Geometry check sheet. Reference: the model listing, model coordinates, mm. Face numbers are marked on the shaded views. A direction names the side the tool comes from. Give positions to 0.01 mm unless a question says otherwise; leave off trailing zeros. Order: outer loops, then holes, each group sorted by start corner. A loop starts at its lowest first (then second) coordinate and runs counter-clockwise, first axis right, second up. Notation, with made-up numbers: M 34.25,-1 L 92.25,-1 A22 cw 92.25,12 Z; hole C 38.5,-29 d6. An arc over 180 degrees is marked long. Put each result on its own line as item: value. Start each with the question number.
Q1. Material ranges on L1, parallel to X at y = -2.8, z = -135.5; L2, parallel to Z at x = 66.5, y = -4.25; L3, parallel to X at y = -14, z = -90, recorded low to high.
Q2. Section check B-B on z = -128.5. Record the cut outline in (x, y), then the cut area to 3 significant figures.
Q3. Access from +Z, -Z, +X, -X, +Y, -Y to the whole of each face (thin tool, end or side, straight path). Record for the marked faces 3 and 4.
Q4. Section check A-A on y = -12.5. Record the cut outline in (x, z).
Q5. Go/stop test with flat-tipped pins: pin 1 (1.6 mm diameter, centred on y = 1, z = -13.5, fed in from +X); pin 2 (3.5 mm diameter, centred on x = 94.5, z = -21, fed in from -Y); pin 3 (3.5 mm diameter, centred on x = 185, z = -22.5, fed in from -Y). Record where each tip stops, or that it passes through.
Q6. Mould release check, pull along X, two halves, no side actions. Record for the marked faces 1 and 2: +X half, -X half, draft (parallel to the pull), parting line (faces both ways), or undercut.
Q7. Section check C-C on z = -33. Record the cut outline in (x, y), then the cut area to 3 significant figures.
```python
from build123d import *

# Parameters (mm, degrees)
BOSS_EXTRUDE1_DEPTH     = 2
SKETCH2_W               = 45
SKETCH2_H               = 5
BOSS_EXTRUDE2_DEPTH     = 10
BOSS_EXTRUDE3_DEPTH     = 20
SKETCH4_W               = 67
SKETCH4_H               = 2
BOSS_EXTRUDE4_DEPTH     = 5
SKETCH5_W               = 58
SKETCH5_H               = 72.3
SKETCH5_W_2             = 55
SKETCH5_H_2             = 69.3
BOSS_EXTRUDE5_DEPTH     = 19
SKETCH6_W               = 13
SKETCH6_H               = 13
SKETCH6_W_2             = 10
CUT_EXTRUDE1_DEPTH      = 1.5
BOSS_EXTRUDE6_DEPTH     = 10
CUT_EXTRUDE2_START      = -6
SKETCH9_W               = 45
SKETCH9_H               = 1.5
CUT_EXTRUDE2_DEPTH      = 7
CUT_EXTRUDE3_DEPTH      = 12
SKETCH11_R              = 2.5
SKETCH11_R_2            = 1.5
BOSS_EXTRUDE7_DEPTH     = 4
SKETCH12_W              = 34
SKETCH12_H              = 63
SKETCH12_W_2            = 32
SKETCH12_H_2            = 61
BOSS_EXTRUDE8_DEPTH     = 4
SKETCH13_W              = 8
SKETCH13_H              = 4
CUT_EXTRUDE4_DEPTH      = 18
SKETCH14_R              = 6
SKETCH14_W              = 64
SKETCH14_H              = 39
CUT_EXTRUDE5_DEPTH      = 21
CUT_EXTRUDE5_DEPTH_BACK = 3
SKETCH15_W              = 100
SKETCH15_H              = 3
SKETCH15_W_2            = 112
BOSS_EXTRUDE9_DEPTH     = 5
CUT_EXTRUDE6_DEPTH      = 5


with BuildPart() as part:
    # Sketch1 → Boss-Extrude1 (new body)
    with BuildSketch(Plane(origin=(0, 0, 0), x_dir=(1, 0, 0), z_dir=(0, 1, 0))):
        with BuildLine():
            Line((124.25, 158), (176, 158))
            ThreePointArc((176, 158), (189.435028843, 152.435028843), (195, 139))
            Line((195, 139), (195, 19))
            ThreePointArc((195, 19), (189.435028843, 5.564971157), (176, 0))
            Line((176, 0), (162, 0))
            Line((162, 0), (162, 17))
            Line((162, 17), (120, 17))
            Line((120, 17), (120, 0))
            Line((120, 0), (75, 0))
            Line((75, 0), (75, 17))
            Line((75, 17), (33, 17))
            Line((33, 17), (33, 0))
            Line((33, 0), (19, 0))
            ThreePointArc((19, 0), (5.564971157, 5.564971157), (0, 19))
            Line((0, 19), (0, 139))
            ThreePointArc((0, 139), (5.564971157, 152.435028843), (19, 158))
            Line((19, 158), (70.75, 158))
            Line((70.75, 158), (70.75, 143))
            Line((70.75, 143), (80.75, 143))
            Line((80.75, 143), (80.75, 88))
            Line((80.75, 88), (114.25, 88))
            Line((114.25, 88), (114.25, 143))
            Line((114.25, 143), (124.25, 143))
            Line((124.25, 143), (124.25, 158))
        make_face()
    extrude(amount=BOSS_EXTRUDE1_DEPTH)

    # Sketch2 → Boss-Extrude2 (add)
    with BuildSketch(Plane.XZ):
        with Locations((97.5, -2.5)):
            Rectangle(SKETCH2_W, SKETCH2_H)
        with BuildLine():
            Line((33, 0), (33, -5))
            Line((33, -5), (19, -5))
            ThreePointArc((19, -5), (9.100505063, -9.100505063), (5, -19))
            Line((5, -19), (5, -139))
            ThreePointArc((5, -139), (9.100505063, -148.899494937), (19, -153))
            Line((19, -153), (70.75, -153))
            Line((70.75, -153), (70.75, -158))
            Line((70.75, -158), (19, -158))
            ThreePointArc((19, -158), (5.564971157, -152.435028843), (0, -139))
            Line((0, -139), (0, -19))
            ThreePointArc((0, -19), (5.564971157, -5.564971157), (19, 0))
            Line((19, 0), (33, 0))
        make_face()
        with BuildLine():
            Line((162, 0), (162, -5))
            Line((162, -5), (176, -5))
            ThreePointArc((176, -5), (185.899494937, -9.100505063), (190, -19))
            Line((190, -19), (190, -139))
            ThreePointArc((190, -139), (185.899494937, -148.899494937), (176, -153))
            Line((176, -153), (124.25, -153))
            Line((124.25, -153), (124.25, -158))
            Line((124.25, -158), (176, -158))
            ThreePointArc((176, -158), (189.435028843, -152.435028843), (195, -139))
            Line((195, -139), (195, -19))
            ThreePointArc((195, -19), (189.435028843, -5.564971157), (176, 0))
            Line((176, 0), (162, 0))
        make_face()
    extrude(amount=BOSS_EXTRUDE2_DEPTH)

    # Sketch3 → Boss-Extrude3 (add)
    with BuildSketch(Plane.XZ):
        Polygon((190, -43.5), (150, -43.5), (150, -114.5), (190, -114.5), (190, -112.5), (152, -112.5), (152, -45.5), (190, -45.5), align=None)
    extrude(amount=BOSS_EXTRUDE3_DEPTH)

    # Sketch4 → Boss-Extrude4 (add)
    with BuildSketch(Plane(origin=(152, 0, 0), x_dir=(0, 0, -1), z_dir=(1, 0, 0))):
        with Locations((79, -19)):
            Rectangle(SKETCH4_W, SKETCH4_H)
    extrude(amount=BOSS_EXTRUDE4_DEPTH)

    # Sketch5 → Boss-Extrude5 (add)
    with BuildSketch(Plane.XZ):
        with Locations((41.75, -116.85)):
            Rectangle(SKETCH5_W, SKETCH5_H)
        with Locations((41.75, -116.85)):
            Rectangle(SKETCH5_W_2, SKETCH5_H_2, mode=Mode.SUBTRACT)
    extrude(amount=BOSS_EXTRUDE5_DEPTH)

    # Sketch6 → Cut-Extrude1 (cut)
    with BuildSketch(Plane.XY.offset(-80.7)):
        with Locations((52.25, -9.5)):
            Rectangle(SKETCH6_W, SKETCH6_H)
        with Locations((20.75, -9.5)):
            Rectangle(SKETCH6_W_2, SKETCH6_H)
    extrude(amount=-CUT_EXTRUDE1_DEPTH, mode=Mode.SUBTRACT)

    # Sketch8 → Boss-Extrude6 (add, symmetric)
    with BuildSketch(Plane(origin=(29.25, 0, 0), x_dir=(0, 0, -1), z_dir=(1, 0, 0))):
        Polygon((151.5, -3.5), (150.5, -3.5), (151.5, -9.5), align=None)
    extrude(amount=BOSS_EXTRUDE6_DEPTH, both=True)

    # Sketch9 → Cut-Extrude2 (cut, through all)
    with BuildSketch(Plane.XZ.offset(10).offset(CUT_EXTRUDE2_START)):
        with BuildLine():
            ThreePointArc((0, -139), (5.564971157, -152.435028843), (19, -158))
            Line((19, -158), (70.75, -158))
            Line((70.75, -158), (70.75, -156.5))
            Line((70.75, -156.5), (19, -156.5))
            ThreePointArc((19, -156.5), (6.625631329, -151.374368671), (1.5, -139))
            Line((1.5, -139), (1.5, -19))
            ThreePointArc((1.5, -19), (6.625631329, -6.625631329), (19, -1.5))
            Line((19, -1.5), (33, -1.5))
            Line((33, -1.5), (33, 0))
            Line((33, 0), (19, 0))
            ThreePointArc((19, 0), (5.564971157, -5.564971157), (0, -19))
            Line((0, -19), (0, -139))
        make_face()
        with BuildLine():
            ThreePointArc((193.5, -19), (188.374368671, -6.625631329), (176, -1.5))
            Line((176, -1.5), (162, -1.5))
            Line((162, -1.5), (162, 0))
            Line((162, 0), (176, 0))
            ThreePointArc((176, 0), (189.435028843, -5.564971157), (195, -19))
            Line((195, -19), (195, -139))
            ThreePointArc((195, -139), (189.435028843, -152.435028843), (176, -158))
            Line((176, -158), (124.25, -158))
            Line((124.25, -158), (124.25, -156.5))
            Line((124.25, -156.5), (176, -156.5))
            ThreePointArc((176, -156.5), (188.374368671, -151.374368671), (193.5, -139))
            Line((193.5, -139), (193.5, -19))
        make_face()
        with Locations((97.5, -0.75)):
            Rectangle(SKETCH9_W, SKETCH9_H)
    extrude(amount=-CUT_EXTRUDE2_DEPTH, mode=Mode.SUBTRACT)

    # Sketch10 → Cut-Extrude3 (cut)
    with BuildSketch(Plane(origin=(0, 2, 0), x_dir=(1, 0, 0), z_dir=(0, 1, 0))):
        with BuildLine():
            Line((176, 0), (19, 0))
            ThreePointArc((19, 0), (8.54772752, 3.133368347), (1.54290975, 11.5))
            Line((1.54290975, 11.5), (193.45709025, 11.5))
            ThreePointArc((193.45709025, 11.5), (186.45227248, 3.133368347), (176, 0))
        make_face()
    extrude(amount=-CUT_EXTRUDE3_DEPTH, mode=Mode.SUBTRACT)

    # Sketch11 → Boss-Extrude7 (add)
    with BuildSketch(Plane.XZ):
        with Locations(Location((185, -119.5, 0), (0, 0, 90))):  # turned: the seam where the file's is
            Circle(SKETCH11_R)
        with Locations(Location((185, -119.5, 0), (0, 0, 270))):  # turned: the seam where the file's is
            Circle(SKETCH11_R_2, mode=Mode.SUBTRACT)
        with Locations(Location((185, -135.5, 0), (0, 0, 90))):  # turned: the seam where the file's is
            Circle(SKETCH11_R)
        with Locations(Location((185, -135.5, 0), (0, 0, 270))):  # turned: the seam where the file's is
            Circle(SKETCH11_R_2, mode=Mode.SUBTRACT)
        with Locations(Location((185, -38.5, 0), (0, 0, 90))):  # turned: the seam where the file's is
            Circle(SKETCH11_R)
        with Locations(Location((185, -38.5, 0), (0, 0, 90))):  # turned: the seam where the file's is
            Circle(SKETCH11_R_2, mode=Mode.SUBTRACT)
        with Locations(Location((185, -22.5, 0), (0, 0, 90))):  # turned: the seam where the file's is
            Circle(SKETCH11_R)
        with Locations(Location((185, -22.5, 0), (0, 0, 90))):  # turned: the seam where the file's is
            Circle(SKETCH11_R_2, mode=Mode.SUBTRACT)
    extrude(amount=BOSS_EXTRUDE7_DEPTH)

    # Sketch12 → Boss-Extrude8 (add)
    with BuildSketch(Plane.XZ):
        with Locations((21, -48.5)):
            Rectangle(SKETCH12_W, SKETCH12_H)
        with Locations((21, -48.5)):
            Rectangle(SKETCH12_W_2, SKETCH12_H_2, mode=Mode.SUBTRACT)
    extrude(amount=BOSS_EXTRUDE8_DEPTH)

    # Sketch13 → Cut-Extrude4 (cut)
    with BuildSketch(Plane(origin=(5, 0, 0), x_dir=(0, 0, -1), z_dir=(1, 0, 0))):
        with Locations((67, -4)):
            Rectangle(SKETCH13_W, SKETCH13_H)
    extrude(amount=-CUT_EXTRUDE4_DEPTH, mode=Mode.SUBTRACT)

    # Sketch14 → Cut-Extrude5 (cut, two sides)
    with BuildSketch(Plane.XZ) as cut_extrude5_sk:
        with Locations(Location((97.5, -78, 0), (0, 0, 270))):  # turned: the seam where the file's is
            Circle(SKETCH14_R)
        with Locations((97.5, -43.5)):
            Rectangle(SKETCH14_W, SKETCH14_H)
    extrude(amount=CUT_EXTRUDE5_DEPTH, mode=Mode.SUBTRACT)
    extrude(cut_extrude5_sk.sketch, amount=-CUT_EXTRUDE5_DEPTH_BACK, mode=Mode.SUBTRACT)

    # Sketch15 → Boss-Extrude9 (add)
    with BuildSketch(Plane.XZ):
        with Locations((97.5, -20.5)):
            Rectangle(SKETCH15_W, SKETCH15_H)
        with Locations((94, -66.5)):
            Rectangle(SKETCH15_W_2, SKETCH15_H)
    extrude(amount=BOSS_EXTRUDE9_DEPTH)

    # Sketch16 → Cut-Extrude6 (cut)
    with BuildSketch(Plane(origin=(0, 0, -22), x_dir=(-1, 0, 0), z_dir=(0, 0, -1))):
        Polygon((-47.5, 0), (-56.160254038, -5), (-47.5, -5), align=None)
        Polygon((-147.5, 0), (-138.839745962, -5), (-147.5, -5), align=None)
    extrude(amount=-CUT_EXTRUDE6_DEPTH, mode=Mode.SUBTRACT)


solid = part.part
```
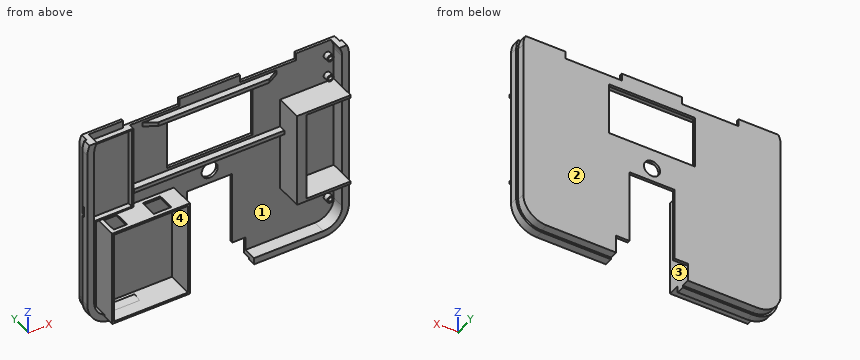
Results found:
1. L1: x = 1.5 to 5, 12.75 to 14.25, 69.25 to 70.75, 182.5 to 183.5, 186.5 to 187.5, 190 to 193.5
1. L2: z = -158 to -151.5, -82.2 to -80.7, -68 to -65, -22 to -19
1. L3: x = 12.75 to 14.25, 69.25 to 70.75, 150 to 152
2. outline: M 0,-10 L 5,-10 L 5,0 L 12.75,0 L 12.75,-19 L 14.25,-19 L 14.25,0 L 69.25,0 L 69.25,-19 L 70.75,-19 L 70.75,0 L 80.75,0 L 80.75,2 L 1.5,2 L 1.5,-4 L 0,-4 Z; M 114.25,0 L 190,0 L 190,-10 L 195,-10 L 195,-4 L 193.5,-4 L 193.5,2 L 114.25,2 Z
2. area: 462 mm^2
3. face 3: -Z, -Y
3. face 4: -Y
4. outline: M 12.75,-153 L 70.75,-153 L 70.75,-80.7 L 58.75,-80.7 L 58.75,-82.2 L 69.25,-82.2 L 69.25,-151.5 L 14.25,-151.5 L 14.25,-82.2 L 15.75,-82.2 L 15.75,-80.7 L 12.75,-80.7 Z; M 25.75,-82.2 L 45.75,-82.2 L 45.75,-80.7 L 25.75,-80.7 Z; M 150,-114.5 L 190,-114.5 L 190,-112.5 L 152,-112.5 L 152,-45.5 L 190,-45.5 L 190,-43.5 L 150,-43.5 Z
5. pin 1: stops at x = 192.86
5. pin 2: stops at y = -5
5. pin 3: stops at y = -4
6. face 1: undercut
6. face 2: draft
7. outline: M 0,-10 L 5,-10 L 5,0 L 37,0 L 37,-4 L 38,-4 L 38,0 L 65.5,0 L 65.5,2 L 1.5,2 L 1.5,-4 L 0,-4 Z; M 129.5,0 L 190,0 L 190,-10 L 195,-10 L 195,-4 L 193.5,-4 L 193.5,2 L 129.5,2 Z
7. area: 348 mm^2
